from build123d import *

# Parameters (mm, degrees)
BOSS_EXTRUDE1_DEPTH        = 38.1
F_8_0_199_DIAMETER_HOLE1_D = 5.0546
CUT_EXTRUDE1_START         = -3.175
CUT_EXTRUDE1_OUTLINE_R     = 6.350000009
CUT_EXTRUDE1_DEPTH         = 3.175
M3_CLEARANCE_HOLE1_D       = 3.4


# Read off the part's stored shape, not the designer's step: Cut-Extrude1
with BuildPart() as part:
    # Sketch1 → Boss-Extrude1 (new body)
    with BuildSketch(Plane(origin=(0, 0, 0), x_dir=(0, 0, -1), z_dir=(1, 0, 0))):
        with BuildLine():
            Line((0, 42.094372261), (0, 6.675328802))
            ThreePointArc((0, 6.675328802), (0.785233991, 4.779606252), (2.680956542, 3.994372261))
            Line((2.680956542, 3.994372261), (45.085, 3.994372261))
            ThreePointArc((45.085, 3.994372261), (46.881051224, 3.250423485), (47.625, 1.454372261))
            Line((47.625, 1.454372261), (47.625, -11.880627739))
            Line((47.625, -11.880627739), (44.45, -11.880627739))
            Line((44.45, -11.880627739), (44.45, -1.720627739))
            ThreePointArc((44.45, -1.720627739), (43.706051224, 0.075423485), (41.91, 0.819372261))
            Line((41.91, 0.819372261), (-0.494043458, 0.819372261))
            ThreePointArc((-0.494043458, 0.819372261), (-2.389766009, 1.604606252), (-3.175, 3.500328802))
            Line((-3.175, 3.500328802), (-3.175, 42.094372261))
            Line((-3.175, 42.094372261), (0, 42.094372261))
        make_face()
    extrude(amount=BOSS_EXTRUDE1_DEPTH)

    # 8 _0.199_ Diameter Hole1 (through all)
    with Locations(Plane.XY.offset(-44.45)):
        with Locations((7.9375, -7.118127739), (30.1625, -7.118127739)):
            Hole(F_8_0_199_DIAMETER_HOLE1_D / 2)

    # Cut-Extrude1 outline → Cut-Extrude1 (cut)
    with BuildSketch(Plane.XY.offset(3.175).offset(CUT_EXTRUDE1_START)):
        with BuildLine():
            ThreePointArc((0, 23.044372261), (5.579615818, 36.514756443), (19.05, 42.094372261))
            Line((19.05, 42.094372261), (0, 42.094372261))
            Line((0, 42.094372261), (0, 23.044372261))
        make_face()
        with BuildLine():
            ThreePointArc((19.05, 42.094372261), (32.520384182, 36.514756443), (38.1, 23.044372261))
            Line((38.1, 23.044372261), (38.1, 42.094372261))
            Line((38.1, 42.094372261), (19.05, 42.094372261))
        make_face()
        with Locations((19.05, 30.044372231)):
            Circle(CUT_EXTRUDE1_OUTLINE_R)
    extrude(amount=CUT_EXTRUDE1_DEPTH, mode=Mode.SUBTRACT)

    # M3 Clearance Hole1 (through all)
    with Locations(Plane.XY.offset(3.175)):
        with Locations((3.55, 23.044372261), (34.55, 23.044372261), (26.8, 9.620978502), (11.3, 9.620978502)):
            Hole(M3_CLEARANCE_HOLE1_D / 2)


solid = part.part
The listing builds one solid part. Answer for the finished solid, in the listing's coordinates (mm). A direction names the side the tool comes from. Give positions to 0.01 mm unless a question says otherwise; leave off trailing zeros. Loops run counter-clockwise (first coordinate to the right, second up) from the corner with the lowest first, then second, coordinate; pieces in that order, holes last. Notation, with made-up numbers: (76.5, 79.5) - (104.5, 79.5) arc R12 ccw to (104.5, 98.5) - close; hole circle Ø11 at (43.25, 55.25). An arc over 180 degrees is marked (long way). Write each question's results on one line, items separated by ' | '.
1. For a pull along Y with two mould halves and no side action, classify faces 1 (the face through (18.78, 3.27, -46.86)), 2 (the face through (19, 23, 3.175)), 3 (the face through (5.527, -6.359, -46.06)) as +Y half, -Y half, draft (parallel to the pull), parting line (faces both ways), or undercut.
Resolved:
face 1: +Y half | face 2: draft | face 3: undercut
2. Find section B-B, the plane z = -5. Write down the section's boundary in (x, y), then the cut area to 3 significant figures.
Resolved:
outline: (0, 0.82) - (38.1, 0.82) - (38.1, 3.99) - (0, 3.99) - close | area: 121 mm^2
3. Which of the six approach directions +Z, -Z, +X, -X, +Y, -Y give full straight-line access (tool end or side, diameter ignored) to faces 4 (the face through (19, 3.994, -24)), 5 (the face through (18.22, 36.34, 1.57)), 6 (the face through (19, -7, -44.45))?
Resolved:
face 4: -Z, +X, -X, +Y | face 5: +Z, -Z | face 6: +Z, +X, -X, -Y
4. Flat-ended cylindrical pins translate along their axes: P1, Ø20.5, axis at x = 19.05, y = 30.04, coming from the -Z side; P2, Ø2.5, axis at x = 11.3, y = 9.62, coming from the +Z side; P3, Ø4, axis at x = 10, z = -24, coming from the +Y side; P4, Ø19, axis at x = 16.5, z = -13, coming from the -Y side. Find the tip coordinate at first contact, or state that the pin passes through.
Resolved:
P1: stops at z = 0 | P2: passes through | P3: stops at y = 3.99 | P4: stops at y = 0.82
5. Consider probe 1 along Z at (x, y) = (20, 22) (3 decimals); probe 2 along Y at (x, z) = (3.55, 2.3); probe 3 along Z at (x, y) = (26.5, -7.5) (3 decimals). Determine where each line is inside the solid, lowest interval first. Write a range as from..to.
Resolved:
probe 1: z = 0..3.175 | probe 2: y = 1.52..21.34, 24.74..34.12 | probe 3: z = -47.625..-44.45
6. Find section A-A, the plane x = 3.55. Write down the section's boundary in (y, z) (3 decimals), then the cut area to 3 significant figures.
Resolved:
outline: (-11.881, -47.625) - (1.454, -47.625) arc R2.54 ccw to (3.994, -45.085) - (3.994, -2.681) arc R2.681 cw to (6.675, 0) - (21.344, 0) - (21.344, 3.175) - (3.5, 3.175) arc R2.681 ccw to (0.819, 0.494) - (0.819, -41.91) arc R2.54 cw to (-1.721, -44.45) - (-11.881, -44.45) - close; (24.744, 0) - (34.119, 0) - (34.119, 3.175) - (24.744, 3.175) - close | area: 286 mm^2
7. Find section D-D, the plane y = 20. Write down the section's boundary in (x, z) (3 decimals), then the cut area to 3 significant figures.
Resolved:
outline: (0, 0) - (38.1, 0) - (38.1, 3.175) - (0, 3.175) - close | area: 121 mm^2
8. Find section C-C, the plane x = 22.5. Write down the section's boundary in (y, z) (3 decimals), then the cut area to 3 significant figures.
Resolved:
outline: (-11.881, -47.625) - (1.454, -47.625) arc R2.54 ccw to (3.994, -45.085) - (3.994, -2.681) arc R2.681 cw to (6.675, 0) - (24.713, 0) - (24.713, 3.175) - (3.5, 3.175) arc R2.681 ccw to (0.819, 0.494) - (0.819, -41.91) arc R2.54 cw to (-1.721, -44.45) - (-11.881, -44.45) - close; (35.375, 0) - (41.779, 0) - (41.779, 3.175) - (35.375, 3.175) - close | area: 288 mm^2
